Geometry check sheet. Reference: drawing and pictorial views, mm from the part's lowest x, y, z. Coordinates: 2 decimals unless noted, no trailing zeros. Write each loop counter-clockwise with the first axis right and the second up, starting at its lowest first coordinate (ties: lowest second). Pieces come first, ordered by that corner, then holes. Notation, with made-up numbers: (68, -19.75) -> (112, -19.75) arc R38 cw to (112, 18.25) -> close; hole circle Ø6 at (31, -12). An arc over 180 degrees is marked (long way). Answer in a Markdown table with one row per item.
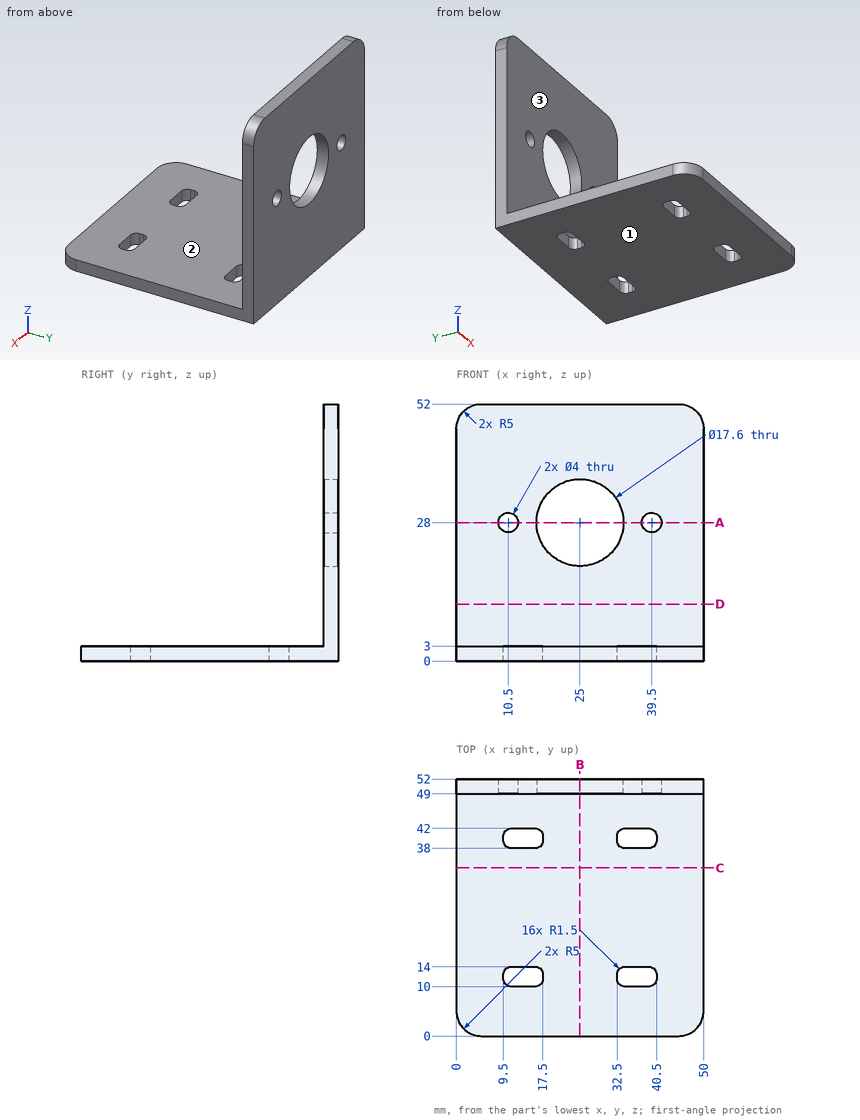
1. Section check D-D, the plane z = 11.5. Record the boundary of the cut face in (x, y).
Geometry says:
| item | result |
|---|---|
| outline | (0, 49) -> (50, 49) -> (50, 52) -> (0, 52) -> close |
2. Section check B-B, the plane x = 25. Record the boundary of the cut face in (y, z), plus the area to 3 significant figures.
Geometry says:
| item | result |
|---|---|
| outline | (0, 0) -> (52, 0) -> (52, 19.2) -> (49, 19.2) -> (49, 3) -> (0, 3) -> close; (49, 36.8) -> (52, 36.8) -> (52, 52) -> (49, 52) -> close |
| area | 250 mm^2 |
3. Mould release check, pull along Z, two halves, no side actions. Record for the marked faces 1, 2 and 3: released by +Z, released by -Z, zero draft, split by the parting line, or undercut.
Geometry says:
| item | result |
|---|---|
| face 1 | released by -Z |
| face 2 | released by +Z |
| face 3 | zero draft |
4. Thickness scan on line 1 (Y direction, x = 39, z = 23.5); line 2 (Z direction, x = 10.5, y = 50); line 3 (Z direction, x = 39, y = 51). Record the ranges inside material, lowest first. Write a range as from..to.
Geometry says:
| item | result |
|---|---|
| line 1 | 49..52 |
| line 2 | 0..26, 30..52 |
| line 3 | 0..26.06, 29.94..52 |
5. Depth check by flat-ended pin: P1, Ø6.5, axis at x = 10.5, z = 28, coming from the -Y side; P2, Ø24.5, axis at x = 33, y = 16, coming from the +Z side. Enter the tip coordinate at first touch or a pass-through.
Geometry says:
| item | result |
|---|---|
| P1 | y = 49 |
| P2 | z = 3 |
6. Section check C-C, the plane y = 34. Record the boundary of the cut face in (x, z).
Geometry says:
| item | result |
|---|---|
| outline | (0, 0) -> (50, 0) -> (50, 3) -> (0, 3) -> close |
7. Section check A-A, the plane z = 28. Record the boundary of the cut face in (x, y).
Geometry says:
| item | result |
|---|---|
| outline | (0, 49) -> (8.5, 49) -> (8.5, 52) -> (0, 52) -> close; (12.5, 49) -> (16.2, 49) -> (16.2, 52) -> (12.5, 52) -> close; (33.8, 49) -> (37.5, 49) -> (37.5, 52) -> (33.8, 52) -> close; (41.5, 49) -> (50, 49) -> (50, 52) -> (41.5, 52) -> close |
